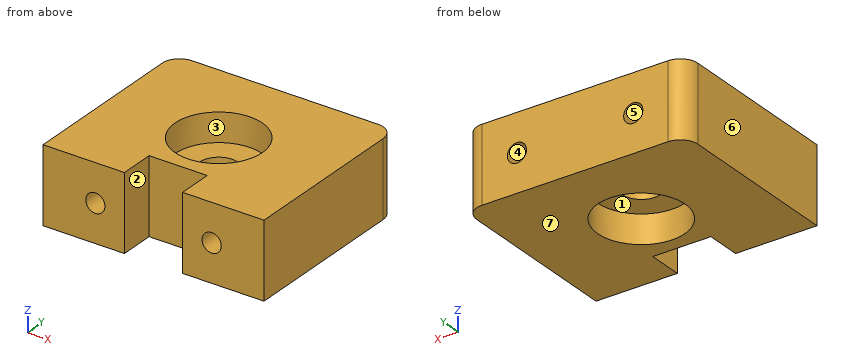
from build123d import *

# Parameters (mm, degrees)
SKETCH1_R                 = 7.5
BOSS_EXTRUDE1_DEPTH       = 13
SKETCH3_R                 = 8.7376
SKETCH3_R_2               = 3.27025
BOSS_EXTRUDE2_DEPTH       = 1.5875
BOSS_EXTRUDE2_DEPTH_BACK  = 1.5875
M4X0_7_TAPPED_HOLE1_D     = 3.3
M4X0_7_TAPPED_HOLE1_DEPTH = 10.1092
M4X0_7_TAPPED_HOLE1_TIP   = 0.991420021
M4X0_7_TAPPED_HOLE2_D     = 3.3
M4X0_7_TAPPED_HOLE2_DEPTH = 10
M4X0_7_TAPPED_HOLE2_TIP   = 0.991420021
SKETCH11_W                = 10
SKETCH11_H                = 6
CUT_EXTRUDE1_DEPTH        = 15


with BuildPart() as part:
    # Sketch1 → Boss-Extrude1 (new body)
    with BuildSketch(Plane.XY):
        with BuildLine():
            Line((-16, 32), (16, 32))
            ThreePointArc((16, 32), (18.121320344, 31.121320344), (19, 29))
            Line((19, 29), (19, 0))
            Line((19, 0), (0, 0))
            Line((0, 0), (-19, 0))
            Line((-19, 0), (-19, 29))
            ThreePointArc((-19, 29), (-18.121320344, 31.121320344), (-16, 32))
        make_face()
        with Locations((0, 15.874)):
            Circle(SKETCH1_R, mode=Mode.SUBTRACT)
    extrude(amount=BOSS_EXTRUDE1_DEPTH)

    # Sketch3 → Boss-Extrude2 (add, two sides)
    with BuildSketch(Plane.XY.offset(6.5)) as boss_extrude2_sk:
        with Locations((0, 15.874)):
            Circle(SKETCH3_R)
        with Locations((0, 15.874)):
            Circle(SKETCH3_R_2, mode=Mode.SUBTRACT)
    extrude(amount=BOSS_EXTRUDE2_DEPTH)
    extrude(boss_extrude2_sk.sketch, amount=-BOSS_EXTRUDE2_DEPTH_BACK)

    # M4x0.7 Tapped Hole1
    with Locations(Plane(origin=(0, 0, 0), x_dir=(-1, 0, 0), z_dir=(0, -1, 0))):
        with Locations((10, -6.5), (-10, -6.5)):
            Hole(M4X0_7_TAPPED_HOLE1_D / 2, depth=M4X0_7_TAPPED_HOLE1_DEPTH)
            with Locations((0, 0, -(M4X0_7_TAPPED_HOLE1_DEPTH + M4X0_7_TAPPED_HOLE1_TIP / 2))):  # 118° drill point
                Cone(0, M4X0_7_TAPPED_HOLE1_D / 2, M4X0_7_TAPPED_HOLE1_TIP, mode=Mode.SUBTRACT)

    # M4x0.7 Tapped Hole2
    with Locations(Plane(origin=(0, 32, 0), x_dir=(1, 0, 0), z_dir=(0, 1, 0))):
        with Locations((-10, -6.5), (10, -6.5)):
            Hole(M4X0_7_TAPPED_HOLE2_D / 2, depth=M4X0_7_TAPPED_HOLE2_DEPTH)
            with Locations((0, 0, -(M4X0_7_TAPPED_HOLE2_DEPTH + M4X0_7_TAPPED_HOLE2_TIP / 2))):  # 118° drill point
                Cone(0, M4X0_7_TAPPED_HOLE2_D / 2, M4X0_7_TAPPED_HOLE2_TIP, mode=Mode.SUBTRACT)

    # Sketch11 → Cut-Extrude1 (cut)
    with BuildSketch(Plane.XY.offset(13)):
        with Locations((0, 3)):
            Rectangle(SKETCH11_W, SKETCH11_H)
    extrude(amount=-CUT_EXTRUDE1_DEPTH, mode=Mode.SUBTRACT)


solid = part.part
Geometry: final body of the model. Coordinates: model frame, mm. Face numbers are marked on the shaded views. A direction names the side the tool comes from. Give positions to 0.01 mm unless a question says otherwise; leave off trailing zeros. Order: outer loops, then holes, each group sorted by start corner. A loop starts at its lowest first (then second) coordinate and runs counter-clockwise, first axis right, second up. Notation, with made-up numbers: (10, 50.5) -> (24, 50.5) arc R22 ccw to (24, 65.5) -> close; hole circle Ø7 at (56, -36). An arc over 180 degrees is marked (long way). Put each result on its own line as item: value.
Q1. Material intervals for L1, parallel to X at y = 28.5, z = 6.5; L2, parallel to Z at x = -10, y = 2.5; L3, parallel to Y at x = 0, z = 3.35, sorted ascending.
Here are the results:
L1: x = -19 to -11.65, -8.35 to 8.35, 11.65 to 19
L2: z = 0 to 4.85, 8.15 to 13
L3: y = 6 to 8.37, 23.37 to 32
Q2. Pin query (flat end, axial travel): pin 1 (1 mm diameter, centred on x = 0, y = 25.5, fed in from -Z); pin 2 (2.5 mm diameter, centred on x = 10, z = 6.5, fed in from -Y); pin 3 (8.5 mm diameter, centred on x = 0, y = 15.874, fed in from -Z); pin 4 (2 mm diameter, centred on x = -10, z = 6.5, fed in from +Y). Return the tip coordinate at first contact, or that it passes through.
Here are the results:
pin 1: stops at z = 0
pin 2: stops at y = 10.35
pin 3: stops at z = 4.91
pin 4: stops at y = 21.61
Q3. Draft query along X for the marked faces 5, 6 and 7. Return one class per face: released by +X, released by -X, zero draft, split by the parting line, or undercut.
Here are the results:
face 5: undercut
face 6: released by -X
face 7: zero draft
Q4. Section C-C, the plane z = 9.5. Return loops of the section in (x, y), then the cut area to 3 significant figures.
Here are the results:
outline: (-19, 0) -> (-5, 0) -> (-5, 6) -> (5, 6) -> (5, 0) -> (19, 0) -> (19, 29) arc R3 ccw to (16, 32) -> (-16, 32) arc R3 ccw to (-19, 29) -> close; hole circle Ø15 at (0, 15.87)
area: 975 mm^2
Q5. Section A-A, the plane x = 0. Return loops of the section in (y, z), then the cut area to 3 significant figures.
Here are the results:
outline: (6, 0) -> (8.37, 0) -> (8.37, 4.91) -> (12.6, 4.91) -> (12.6, 8.09) -> (8.37, 8.09) -> (8.37, 13) -> (6, 13) -> close; (19.14, 4.91) -> (23.37, 4.91) -> (23.37, 0) -> (32, 0) -> (32, 13) -> (23.37, 13) -> (23.37, 8.09) -> (19.14, 8.09) -> close
area: 170 mm^2
Q6. Reachability of the marked faces 1, 2, 3 and 4 from +Z, -Z, +X, -X, +Y, -Y: full face, straight path, thin tool, end or side. Return the list, or none.
Here are the results:
face 1: -Z
face 2: +Z, -Z, -Y
face 3: +Z
face 4: +Y
Q7. Section B-B, the plane y = 14. Return loops of the section in (x, z).
Here are the results:
outline: (-19, 0) -> (-7.26, 0) -> (-7.26, 4.91) -> (-2.68, 4.91) -> (-2.68, 8.09) -> (-7.26, 8.09) -> (-7.26, 13) -> (-19, 13) -> close; (2.68, 4.91) -> (7.26, 4.91) -> (7.26, 0) -> (19, 0) -> (19, 13) -> (7.26, 13) -> (7.26, 8.09) -> (2.68, 8.09) -> close
